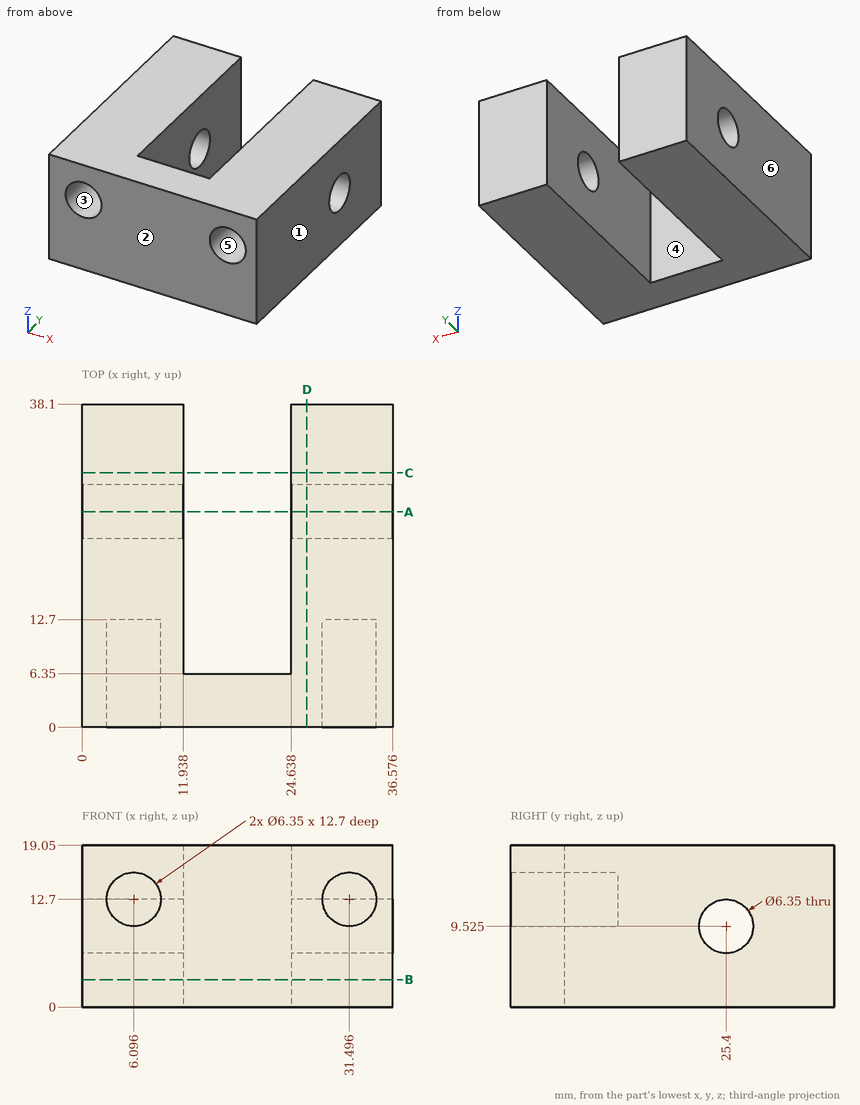
The drawing under review shows one solid part. Ordinate dimensions are in mm from its lowest x, y, z. A direction names the side the tool comes from. Give positions to 0.01 mm unless a question says otherwise; leave off trailing zeros. Write each loop counter-clockwise with the first axis right and the second up, starting at its lowest first coordinate (ties: lowest second). Pieces come first, ordered by that corner, then holes. Notation, with made-up numbers: (9.5, 47) -> (66.5, 47) arc R19 cw to (66.5, 82) -> close; hole circle Ø6 at (83.5, -10.75). An arc over 180 degrees is marked (long way). Answer in a Markdown table with one row per item.
(1) Consider section C-C (y = 30). State the section outline as (x, z) points, then the cut area to 3 significant figures.
Results:
| item | result |
|---|---|
| outline | (0, 0) -> (11.94, 0) -> (11.94, 19.05) -> (0, 19.05) -> close; (24.64, 0) -> (36.58, 0) -> (36.58, 19.05) -> (24.64, 19.05) -> close |
| area | 455 mm2 |
(2) Clearance check with flat-ended pins moving along their axes: pin 1 (6.5 mm diameter, centred on x = 20, z = 10, fed in from +Y); pin 2 (1.9 mm diameter, centred on x = 31, z = 14, fed in from -Y). State where each tip first meets the part, or that it passes through.
Results:
| item | result |
|---|---|
| pin 1 | y = 6.35 |
| pin 2 | y = 12.7 |
(3) Consider section B-B (z = 3.25). State the section outline as (x, y) points, then the cut area to 3 significant figures.
Results:
| item | result |
|---|---|
| outline | (0, 0) -> (36.58, 0) -> (36.58, 38.1) -> (24.64, 38.1) -> (24.64, 6.35) -> (11.94, 6.35) -> (11.94, 38.1) -> (0, 38.1) -> close |
| area | 990 mm2 |
(4) Consider section D-D (x = 26.5). State the section outline as (y, z) points (3 decimals).
Results:
| item | result |
|---|---|
| outline | (0, 0) -> (38.1, 0) -> (38.1, 19.05) -> (0, 19.05) -> close; hole circle Ø6.35 at (25.4, 9.525) |
(5) Mouldability with a two-part tool opening along X and no side actions: class the marked faces 1, 2 and 3 as +X half, -X half, draft (parallel to the pull), parting line (faces both ways), or undercut.
Results:
| item | result |
|---|---|
| face 1 | +X half |
| face 2 | draft |
| face 3 | undercut |
(6) To check wall thickness, follow probe 1 along X at (y, z) = (9.5, 5.25); probe 2 along X at (y, z) = (5.5, 14.5); probe 3 along Z at (x, y) = (11, 24). State the ranges of each line that lie inside material, in increasing order.
Results:
| item | result |
|---|---|
| probe 1 | 0 to 11.94, 24.64 to 36.58 |
| probe 2 | 0 to 3.48, 8.71 to 28.88, 34.11 to 36.58 |
| probe 3 | 0 to 6.68, 12.37 to 19.05 |
(7) For the marked faces 4, 5 and 6, list the 3-axis set-ups (+Z, -Z, +X, -X, +Y, -Y) from which the entire face can be reached by the end or side of a thin tool; tool diameter is ignored.
Results:
| item | result |
|---|---|
| face 4 | +Z, -Z, +Y |
| face 5 | -Y |
| face 6 | +Z, -Z, -X, +Y, -Y |
(8) Consider section A-A (y = 25.4). State the section outline as (x, z) points.
Results:
| item | result |
|---|---|
| outline | (0, 0) -> (11.94, 0) -> (11.94, 6.35) -> (0, 6.35) -> close; (0, 12.7) -> (11.94, 12.7) -> (11.94, 19.05) -> (0, 19.05) -> close; (24.64, 0) -> (36.58, 0) -> (36.58, 6.35) -> (24.64, 6.35) -> close; (24.64, 12.7) -> (36.58, 12.7) -> (36.58, 19.05) -> (24.64, 19.05) -> close |
